Work out the finished part from the listing and answer in its coordinate system (mm). A direction names the side the tool comes from. Round coordinates to 2 decimals unless told otherwise and drop trailing zeros. Loops run counter-clockwise (first coordinate to the right, second up) from the corner with the lowest first, then second, coordinate; pieces in that order, holes last.
Autodesk Inventor part; units mm, degrees
ref_plane "YZ Plane" through (0, 0, 0) normal (1, 0, 0) x (0, 1, 0)
ref_plane "XZ Plane" through (0, 0, 0) normal (0, 1, 0) x (-1, 0, 0)
ref_plane "XY Plane" through (0, 0, 0) normal (0, 0, 1) x (1, 0, 0)
sketch "Náčrt1" plane through (0, 0, 0) normal (0, 0, 1) x (1, 0, 0)
  line L0 (-62.5, 32.5) -> (62.5, 32.5)
  line L1 (62.5, 32.5) -> (62.5, -32.5)
  line L2 (62.5, -32.5) -> (-62.5, -32.5)
  line L3 (-62.5, -32.5) -> (-62.5, 32.5)
  line L4 (-87.5, 0) -> (87.5, 0)
  line L5 (0, 45.5) -> (0, -45.5)
  point P0 (0, 0)
  dimension "d0" = 125
  dimension "d1" = 65
extrude "Vysunutí1" add sketch "Náčrt1" along normal mid plane 50
sketch "Náčrt2" plane through (0, 0, -25) normal (0, 0, -1) x (-1, 0, 0)
  line L0 (-87.5, 0) -> (87.5, 0)
  circle A0 centre (15, 0) radius 27
  line L1 (0, -45.5) -> (0, 45.5)
  dimension "d18" = 54
  dimension "d19" = 15
extrude "Vysunutí2" cut sketch "Náčrt2" against normal blind 10
sketch "Náčrt3" plane through (0, 0, 25) normal (0, 0, 1) x (1, 0, 0)
  line L0 (32.02, 28.5) -> (-51.5, 28.5)
  line L1 (-51.5, 28.5) -> (-51.5, -27.18)
  line L2 (-51.5, -27.18) -> (32.02, -27.18)
  line L3 (32.02, -27.18) -> (32.02, 28.5)
  line L4 (-62.5, 32.5) -> (-62.5, -32.5)
  line L5 (62.5, 32.5) -> (-62.5, 32.5)
  point P0 (0, 0)
  dimension "d8" = 83.52
  dimension "d9" = 55.68
  dimension "d11" = 11
  dimension "d12" = 4
extrude "Vysunutí3" cut sketch "Náčrt3" against normal blind 10
sketch "Náčrt4" plane through (0, 0, -25) normal (0, 0, -1) x (-1, 0, 0)
  line L0 (62.5, -32.5) -> (62.5, 32.5)
  line L1 (62.5, 32.5) -> (-62.5, 32.5)
  line L2 (-62.5, 32.5) -> (-62.5, -32.5)
  line L3 (-62.5, -32.5) -> (62.5, -32.5)
  line L4 (-62.5, 32.5) -> (-32.5, 32.5)
  line L5 (-32.5, 32.5) -> (-32.5, -33.9338)
  line L6 (-32.5, -33.9338) -> (-62.5, -33.9338)
  line L7 (-62.5, -33.9338) -> (-62.5, 32.5)
  point P0 (0, 0)
  point P1 (-32.5, -32.5)
  dimension "d15" = 30
extrude "Vysunutí4" add sketch "Náčrt4" along normal blind 35 contours L3 L2 L1 L5
properties part number "telo1"
1. Find section C-C (x = -15). Write down the section's boundary in (y, z).
Answer key:
outline: (-32.5, -25) - (-27, -25) - (-27, -15) - (27, -15) - (27, -25) - (32.5, -25) - (32.5, 25) - (28.5, 25) - (28.5, 15) - (-27.18, 15) - (-27.18, 25) - (-32.5, 25) - close
2. Determine the mould class of faces 1 (the face through (-62.5, 0, 0)), 2 (the face through (15, -32.5, -7)), 3 (the face through (-51.5, 1, 20)), 4 (the face through (-10, 1, 15)) for opening direction X: +X half, -X half, draft (parallel to the pull), parting line (faces both ways), or undercut.
Answer key:
face 1: -X half
face 2: draft
face 3: undercut
face 4: undercut
3. Find section B-B (y = 0). Write down the section's boundary in (x, z).
Answer key:
outline: (-62.5, -25) - (-42, -25) - (-42, -15) - (12, -15) - (12, -25) - (32.5, -25) - (32.5, -60) - (62.5, -60) - (62.5, 25) - (32.02, 25) - (32.02, 15) - (-51.5, 15) - (-51.5, 25) - (-62.5, 25) - close
4. Find section D-D (z = -22.5). Write down the section's boundary in (x, y), then the cut area to 3 significant figures.
Answer key:
outline: (-62.5, -32.5) - (62.5, -32.5) - (62.5, 32.5) - (-62.5, 32.5) - close; hole circle Ø54 at (-15, 0)
area: 5,830 mm2
5. Consider probe 1 along X at (y, z) = (0, -22); probe 2 along Y at (x, z) = (-29, 19.5); probe 3 along Y at (x, z) = (-15, -23). Determine where each line is inside the solid, lowest interval first.
Answer key:
probe 1: x = -62.5 to -42, 12 to 62.5
probe 2: y = -32.5 to -27.18, 28.5 to 32.5
probe 3: y = -32.5 to -27, 27 to 32.5
6. Which of the six approach directions +Z, -Z, +X, -X, +Y, -Y give full straight-line access (tool end or side, diameter ignored) to faces 5 (the face through (-9.15, -26.36, -20.07)), 6 (the face through (-16, -28, -25)), 7 (the face through (32.02, 0, 20))?
Answer key:
face 5: -Z
face 6: -Z, -X, +Y, -Y
face 7: +Z
7. Given pin 1 (6 mm diameter, centred on x = 9.5, y = -3.5, fed in from +Z); pin 2 (8 mm diameter, centred on x = -38, y = 25, fed in from -Z); pin 3 (16 mm diameter, centred on x = -13.5, y = 12, fed in from -Z), each flat-ended and moving along its own axis, determine where each tip first touches the part or whether it passes through.
Answer key:
pin 1: stops at z = 15
pin 2: stops at z = -25
pin 3: stops at z = -15
8. Find section A-A (z = 19). Write down the section's boundary in (x, y), then the cut area to 3 significant figures.
Answer key:
outline: (-62.5, -32.5) - (62.5, -32.5) - (62.5, 32.5) - (-62.5, 32.5) - close; hole (-51.5, -27.18) - (32.02, -27.18) - (32.02, 28.5) - (-51.5, 28.5) - close
area: 3,470 mm2
